Verification items for the finished model (mm, model axes). A direction names the side the tool comes from. Round coordinates to 2 decimals unless told otherwise and drop trailing zeros. Write each loop counter-clockwise with the first axis right and the second up, starting at its lowest first coordinate (ties: lowest second). Pieces come first, ordered by that corner, then holes. Notation, with made-up numbers: (21, -22) - (40, -22) arc R10 ccw to (40, -14) - close; hole circle Ø7 at (85.5, 46). An arc over 180 degrees is marked (long way). Answer as a JSON object with one key per item and string values. Group by question number.
1) Mould release check, pull along X, two halves, no side actions. Record for faces 1 (the flat face through (-7, -2, 35)), 2 (the flat face through (3, 2, 10)), 3 (the cylindrical face through (-2.17, -9.76, 18.27)): +X half, -X half, draft (parallel to the pull), parting line (faces both ways), or undercut.
2) Thickness scan on line 1 (Y direction, x = 0, z = 8.25); line 2 (Y direction, x = 0, z = 18); line 3 (Z direction, x = 6.25, y = 0.25). Record the ranges inside material, lowest first.
3) Section check D-D (z = 4.5). Enter the section's corners in (x, y).
4) Go/stop test with flat-tipped pins: pin 1 Ø5 at (x, z) = (7.5, 27) entering from +Y; pin 2 Ø1 at (x, z) = (1.5, 29) entering from -Y; pin 3 Ø3 at (x, y) = (1, 1.5) entering from +Z. Record where each tip stops, or that it passes through.
5) Section check A-A (x = 0). Enter the section's corners in (y, z).
6) Section check C-C (z = 22). Enter the section's corners in (x, y), then the cut area to 3 significant figures.
7) Set-up check for faces 4 (the cylindrical face through (6.466, -2.681, 22.675)), 5 (the flat face through (0, 0, 0)): record each of +Z, -Z, +X, -X, +Y, -Y from which the full face is reachable in a straight line by a thin tool's end or side.
```python
from build123d import *

# Parameters (mm, degrees)
F0_R     = 10
F1_DEPTH = 35
F2_R     = 7
F4_DEPTH = 25
F3_R     = 3.25
F5_DEPTH = 30
F6_SIZE  = 2


with BuildPart() as f1:
    # F0 (on Top) → F1 (new body)
    with BuildSketch(Plane.XY):
        Circle(F0_R)
    extrude(amount=F1_DEPTH)

    # F2 (on face) → F4 (cut)
    with BuildSketch(Plane.XY.offset(35)):
        Circle(F2_R)
    extrude(amount=-F4_DEPTH, mode=Mode.SUBTRACT)

    # F3 (on face) → F5 (cut)
    with BuildSketch(Plane.XY.offset(35)):
        Circle(F3_R)
    extrude(amount=-F5_DEPTH, mode=Mode.SUBTRACT)

    # F6
    f6_edges = [f1.edges().sort_by_distance(p)[0] for p in [
        (-10, 0, 0),
    ]]
    chamfer(f6_edges, length=F6_SIZE)


solid = f1.part
```
Returned:
{
 "1": {"face 1": "draft", "face 2": "undercut", "face 3": "parting line"},
 "2": {"line 1": "-10 to -3.25, 3.25 to 10", "line 2": "-10 to -7, 7 to 10", "line 3": "0 to 10"},
 "3": {"outline": "circle Ø20 at (0, 0)"},
 "4": {"pin 1": "y = 8.66", "pin 2": "y = -9.95", "pin 3": "z = 10"},
 "5": {"outline": "(-10, 2) - (-8, 0) - (8, 0) - (10, 2) - (10, 35) - (7, 35) - (7, 10) - (3.25, 10) - (3.25, 5) - (-3.25, 5) - (-3.25, 10) - (-7, 10) - (-7, 35) - (-10, 35) - close"},
 "6": {"outline": "circle Ø20 at (0, 0); hole circle Ø14 at (0, 0)", "area": "160 mm2"},
 "7": {"face 4": "+Z", "face 5": "-Z, +X, -X, +Y, -Y"}
}
